from build123d import *

# Parameters (mm, degrees)
SKETCH1_W            = 42
SKETCH1_H            = 25
BOSS_EXTRUDE1_DEPTH  = 1
SKETCH2_W            = 42
SKETCH2_H            = 1
BOSS_EXTRUDE2_DEPTH  = 179
SKETCH3_W            = 42
SKETCH3_H            = 1
BOSS_EXTRUDE3_DEPTH  = 2.1
SKETCH4_W            = 42
SKETCH4_H            = 1
BOSS_EXTRUDE4_DEPTH  = 15
SKETCH6_R            = 1.25
CUT_EXTRUDE1_DEPTH   = 15
SKETCH7_W            = 42
SKETCH7_H            = 1.67
CUT_EXTRUDE2_DEPTH   = 15
SKETCH8_W            = 8
SKETCH8_H            = 3.5
CUT_EXTRUDE3_DEPTH   = 15
SKETCH9_W            = 42
SKETCH9_H            = 14.33
CUT_EXTRUDE4_DEPTH   = 10
SKETCH10_W           = 5
SKETCH10_H           = 6
BOSS_EXTRUDE5_DEPTH  = 1
SKETCH11_R           = 1
CUT_EXTRUDE5_DEPTH   = 1
SKETCH12_W           = 42
SKETCH12_H           = 1
BOSS_EXTRUDE6_DEPTH  = 9
SKETCH13_W           = 5
SKETCH13_H           = 6
BOSS_EXTRUDE8_DEPTH  = 1
SKETCH15_R           = 1
CUT_EXTRUDE7_DEPTH   = 1
SKETCH16_W           = 6
SKETCH16_H           = 5
BOSS_EXTRUDE9_DEPTH  = 1
SKETCH17_W           = 53
SKETCH17_H           = 5
BOSS_EXTRUDE10_DEPTH = 1
SKETCH18_R           = 1
CUT_EXTRUDE8_DEPTH   = 1
SKETCH20_W           = 1
SKETCH20_H           = 5
BOSS_EXTRUDE11_DEPTH = 1
SKETCH21_R           = 1
CUT_EXTRUDE9_DEPTH   = 1
SKETCH22_W           = 42
SKETCH22_H           = 1
BOSS_EXTRUDE13_DEPTH = 24


with BuildPart() as part:
    # Sketch1 → Boss-Extrude1 (new body)
    with BuildSketch(Plane(origin=(0, 0, 0), x_dir=(1, 0, 0), z_dir=(0, 1, 0))):
        with Locations((4.315789474, -6.763157895)):
            Rectangle(SKETCH1_W, SKETCH1_H)
    extrude(amount=BOSS_EXTRUDE1_DEPTH)

    # Sketch2 → Boss-Extrude2 (add)
    with BuildSketch(Plane(origin=(0, 1, 0), x_dir=(1, 0, 0), z_dir=(0, 1, 0))):
        with Locations((4.315789474, 5.236842105)):
            Rectangle(SKETCH2_W, SKETCH2_H)
    extrude(amount=-BOSS_EXTRUDE2_DEPTH)

    # Sketch3 → Boss-Extrude3 (add)
    with BuildSketch(Plane.XZ.offset(178)):
        with Locations((4.315789474, -5.236842105)):
            Rectangle(SKETCH3_W, SKETCH3_H)
    extrude(amount=BOSS_EXTRUDE3_DEPTH)

    # Sketch4 → Boss-Extrude4 (add)
    with BuildSketch(Plane.XY.offset(-4.736842105)):
        with Locations((4.315789474, -179.6)):
            Rectangle(SKETCH4_W, SKETCH4_H)
    extrude(amount=BOSS_EXTRUDE4_DEPTH)

    # Sketch6 → Cut-Extrude1 (cut)
    with BuildSketch(Plane.XZ.offset(180.1)):
        with Locations((-6.684210526, 3.593157895)):
            Circle(SKETCH6_R)
        with Locations((15.315789474, 3.593157895)):
            Circle(SKETCH6_R)
    extrude(amount=-CUT_EXTRUDE1_DEPTH, mode=Mode.SUBTRACT)

    # Sketch7 → Cut-Extrude2 (cut)
    with BuildSketch(Plane.XZ.offset(180.1)):
        with Locations((4.315789474, 9.428157895)):
            Rectangle(SKETCH7_W, SKETCH7_H)
    extrude(amount=-CUT_EXTRUDE2_DEPTH, mode=Mode.SUBTRACT)

    # Sketch8 → Cut-Extrude3 (cut)
    with BuildSketch(Plane(origin=(0, 1, 0), x_dir=(1, 0, 0), z_dir=(0, 1, 0))):
        with Locations((-12.684210526, -17.513157895)):
            Rectangle(SKETCH8_W, SKETCH8_H)
    extrude(amount=-CUT_EXTRUDE3_DEPTH, mode=Mode.SUBTRACT)

    # Sketch9 → Cut-Extrude4 (cut)
    with BuildSketch(Plane.XZ.offset(180.1)):
        with Locations((4.315789474, 1.428157895)):
            Rectangle(SKETCH9_W, SKETCH9_H)
    extrude(amount=-CUT_EXTRUDE4_DEPTH, mode=Mode.SUBTRACT)

    # Sketch10 → Boss-Extrude5 (add)
    with BuildSketch(Plane(origin=(0, 0, -5.736842105), x_dir=(-1, 0, 0), z_dir=(0, 0, -1))):
        with Locations((-4.315789474, -173.1)):
            Rectangle(SKETCH10_W, SKETCH10_H)
    extrude(amount=-BOSS_EXTRUDE5_DEPTH)

    # Sketch11 → Cut-Extrude5 (cut)
    with BuildSketch(Plane(origin=(0, 0, -5.736842105), x_dir=(-1, 0, 0), z_dir=(0, 0, -1))):
        with Locations((-4.315789474, -173.6)):
            Circle(SKETCH11_R)
    extrude(amount=-CUT_EXTRUDE5_DEPTH, mode=Mode.SUBTRACT)

    # Sketch12 → Boss-Extrude6 (add)
    with BuildSketch(Plane.XZ.offset(170.1)):
        with Locations((4.315789474, -5.236842105)):
            Rectangle(SKETCH12_W, SKETCH12_H)
    extrude(amount=BOSS_EXTRUDE6_DEPTH)

    # Sketch13 → Boss-Extrude8 (add)
    with BuildSketch(Plane(origin=(0, 0, -5.736842105), x_dir=(-1, 0, 0), z_dir=(0, 0, -1))):
        with Locations((-4.315789474, -182.1)):
            Rectangle(SKETCH13_W, SKETCH13_H)
    extrude(amount=-BOSS_EXTRUDE8_DEPTH)

    # Sketch15 → Cut-Extrude7 (cut)
    with BuildSketch(Plane(origin=(0, 0, -5.736842105), x_dir=(-1, 0, 0), z_dir=(0, 0, -1))):
        with Locations((-4.315789474, -182.6)):
            Circle(SKETCH15_R)
    extrude(amount=-CUT_EXTRUDE7_DEPTH, mode=Mode.SUBTRACT)

    # Sketch16 → Boss-Extrude9 (add)
    with BuildSketch(Plane(origin=(0, 0, -5.736842105), x_dir=(-1, 0, 0), z_dir=(0, 0, -1))):
        with Locations((-28.315789474, -89.55)):
            Rectangle(SKETCH16_W, SKETCH16_H)
    extrude(amount=-BOSS_EXTRUDE9_DEPTH)

    # Sketch17 → Boss-Extrude10 (add)
    with BuildSketch(Plane(origin=(0, 0, -5.736842105), x_dir=(-1, 0, 0), z_dir=(0, 0, -1))):
        with Locations((-4.815789474, -89.55)):
            Rectangle(SKETCH17_W, SKETCH17_H)
    extrude(amount=-BOSS_EXTRUDE10_DEPTH)

    # Sketch18 → Cut-Extrude8 (cut)
    with BuildSketch(Plane(origin=(0, 0, -5.736842105), x_dir=(-1, 0, 0), z_dir=(0, 0, -1))):
        with Locations((-28.815789474, -89.55)):
            Circle(SKETCH18_R)
    extrude(amount=-CUT_EXTRUDE8_DEPTH, mode=Mode.SUBTRACT)

    # Sketch20 → Boss-Extrude11 (add)
    with BuildSketch(Plane.ZY.offset(21.684210526)):
        with Locations((-5.236842105, -89.55)):
            Rectangle(SKETCH20_W, SKETCH20_H)
    extrude(amount=BOSS_EXTRUDE11_DEPTH)

    # Sketch21 → Cut-Extrude9 (cut)
    with BuildSketch(Plane(origin=(0, 0, -5.736842105), x_dir=(-1, 0, 0), z_dir=(0, 0, -1))):
        with Locations((20.184210526, -89.55)):
            Circle(SKETCH21_R)
    extrude(amount=-CUT_EXTRUDE9_DEPTH, mode=Mode.SUBTRACT)

    # Sketch22 → Boss-Extrude13 (add)
    with BuildSketch(Plane.XZ.offset(179.1)):
        with Locations((4.315789474, -5.236842105)):
            Rectangle(SKETCH22_W, SKETCH22_H)
    extrude(amount=BOSS_EXTRUDE13_DEPTH)


solid = part.part
Here's how the part is built. I have some questions about the finished solid (model axes, mm). A direction names the side the tool comes from. Coordinates: 2 decimals unless noted, no trailing zeros. Write each loop counter-clockwise with the first axis right and the second up, starting at its lowest first coordinate (ties: lowest second). Pieces come first, ordered by that corner, then holes. Notation, with made-up numbers: (78.5, 48) - (128.5, 48) arc R15 ccw to (128.5, 55) - close; hole circle Ø6 at (71, 65). An arc over 180 degrees is marked (long way). Use one line per item in the form item = value.
1) Suppose I cut it at B-B, the plane z = 4.5. Write out the boundary of the cut face in (x, y), plus the area to 3 significant figures.
Solved:
outline = (-16.68, 0) - (25.32, 0) - (25.32, 1) - (-16.68, 1) - close
area = 42.0 mm2
2) Suppose I cut it at A-A, the plane y = -64.5. Write out the boundary of the cut face in (x, z).
Solved:
outline = (-16.68, -5.74) - (25.32, -5.74) - (25.32, -4.74) - (-16.68, -4.74) - close
3) I need wall thicknesses on line 1 (X direction, y = -89.55, z = -5.25); line 2 (Y direction, x = 6.5, z = -3.75); line 3 (Z direction, x = -15, y = -149). Which ranges of each line are inside material? Lowest first, please.
Solved:
line_1 = -22.68 to -21.18, -19.18 to 27.82, 29.82 to 31.32
line_2 = 0 to 1
line_3 = -5.74 to -4.74
4) I'm going to push flat-ended pins straight in: P1, Ø7, axis at x = -5.5, z = 8.5, coming from the -Y side; P2, Ø1.8, axis at x = -20.18, y = -89.55, coming from the -Z side; P3, Ø6, axis at x = -8.5, y = -24, coming from the +Z side; P4, Ø0.8, axis at y = -173, z = -5.5, coming from the -X side. Where does each tip first touch, or does it pass through?
Solved:
P1 = 0
P2 = through
P3 = -4.74
P4 = -16.68
5) On a 3-axis mill with a long thin cutter (end or side, diameter ignored), from which of +Z, -Z, +X, -X, +Y, -Y can I reach the whole of each face in a straight line? I mean faces 1 (the flat face through (-16.684, -43, -5)), 2 (the flat face through (25.316, -43, -5)), 3 (the flat face through (4, -100, -5.737)), 4 (the flat face through (4, -100, -4.737)). Say none if no direction works.
Solved:
face_1 = +Z, -Z, -X, +Y
face_2 = +Z, -Z, +X, +Y
face_3 = -Z, +X, -X, +Y, -Y
face_4 = +Z, +X, -X, -Y
